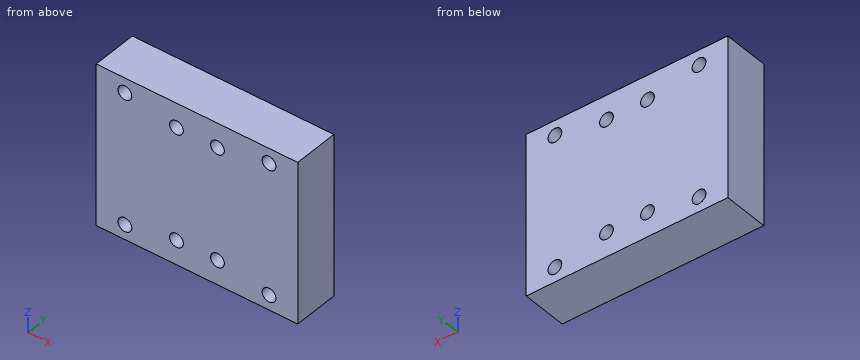
```python
from build123d import *

# Parameters (mm, degrees)
SKETCH1_W                                  = 95.4
SKETCH1_H                                  = 76
BOSS_EXTRUDE1_DEPTH                        = 21.5
SKETCH2_R                                  = 3.25
CUT_EXTRUDE1_DEPTH                         = 22.5
MIRROR1_AT_THE_SECOND_PLANE_COPY_1_SKETC_R = 3.25
MIRROR1_AT_THE_SECOND_PLANE_COPY_1_DEPTH   = 22.5


with BuildPart() as part:
    # Sketch1 → Boss-Extrude1 (new body)
    with BuildSketch(Plane(origin=(0, 0, 0), x_dir=(1, 0, 0), z_dir=(0, 1, 0))):
        Rectangle(SKETCH1_W, SKETCH1_H)
    extrude(amount=BOSS_EXTRUDE1_DEPTH)

    # Sketch2 → Cut-Extrude1 (cut, through all)
    with BuildSketch(Plane(origin=(0, 21.5, 0), x_dir=(1, 0, 0), z_dir=(0, 1, 0))):
        with Locations((-34.1, 31)):
            Circle(SKETCH2_R)
        with Locations((-9.7, 26.5)):
            Circle(SKETCH2_R)
    cut_extrude1 = extrude(amount=-CUT_EXTRUDE1_DEPTH, mode=Mode.SUBTRACT)

    # Mirror1: Cut-Extrude1 across plane
    add(cut_extrude1.mirror(Plane(origin=(0, 0, 0), x_dir=(0, 0, 1), z_dir=(1, 0, 0))), mode=Mode.SUBTRACT)

    # Mirror1 at the second plane: Cut-Extrude1 across plane
    add(cut_extrude1.mirror(Plane.XY), mode=Mode.SUBTRACT)

    # Mirror1 at the second plane copy 1 sketc → Mirror1 at the second plane copy 1 (cut, through all)
    with BuildSketch(Plane(origin=(0, 21.5, 0), x_dir=(-1, 0, 0), z_dir=(0, 1, 0))):
        with Locations((-34.1, 31)):
            Circle(MIRROR1_AT_THE_SECOND_PLANE_COPY_1_SKETC_R)
        with Locations((-9.7, 26.5)):
            Circle(MIRROR1_AT_THE_SECOND_PLANE_COPY_1_SKETC_R)
    extrude(amount=-MIRROR1_AT_THE_SECOND_PLANE_COPY_1_DEPTH, mode=Mode.SUBTRACT)


solid = part.part
```
Source: CAD feature listing. Evaluate the final solid. Frame: model axes, mm. Coordinates: 2 decimals unless noted, no trailing zeros. Order: outer loops, then holes, each group sorted by start corner. A loop starts at its lowest first (then second) coordinate and runs counter-clockwise, first axis right, second up. Notation, with made-up numbers: M 80,7 L 91,7 A18 cw 91,13 Z; hole C -20,-36 d8. An arc over 180 degrees is marked long. Write each question's results on one line, items separated by ' | '. Start each with the question number.
1) Contact query for a flat-ended pin moving along its axis: pin 1 Ø6 at (x, z) = (34.1, 31) entering from -Y. Output: stop coordinate, or through.
2) Section query C-C (z = 31). Return the cut outline in (x, y), plus the area to 3 significant figures.
3) Section query A-A (y = 4.75). Give the number of separate pieces and of enclosed holes in the cut face, plus the area to 3 significant figures.
4) Line query: line 1 (Z direction, x = 9.7, y = 4.5); line 2 (X direction, y = 10, z = -31); line 3 (Z direction, x = 34.1, y = 16). Output: solid intervals per line, ascending. Write a range as from..to.
5) Section query B-B (x = 9.7). Return the cut outline in (y, z), plus the area to 3 significant figures.
Answers:
1) pin 1: passes through
2) outline: M -47.7,0 L -37.35,0 L -37.35,21.5 L -47.7,21.5 Z; M -30.85,0 L 30.85,0 L 30.85,21.5 L -30.85,21.5 Z; M 37.35,0 L 47.7,0 L 47.7,21.5 L 37.35,21.5 Z | area: 1,770 mm^2
3) separate pieces: 1 | enclosed holes: 8 | area: 6,980 mm^2
4) line 1: z = -38..-29.75, -23.25..23.25, 29.75..38 | line 2: x = -47.7..-37.35, -30.85..30.85, 37.35..47.7 | line 3: z = -38..-34.25, -27.75..27.75, 34.25..38
5) outline: M 0,-38 L 21.5,-38 L 21.5,-29.75 L 0,-29.75 Z; M 0,-23.25 L 21.5,-23.25 L 21.5,23.25 L 0,23.25 Z; M 0,29.75 L 21.5,29.75 L 21.5,38 L 0,38 Z | area: 1,350 mm^2
